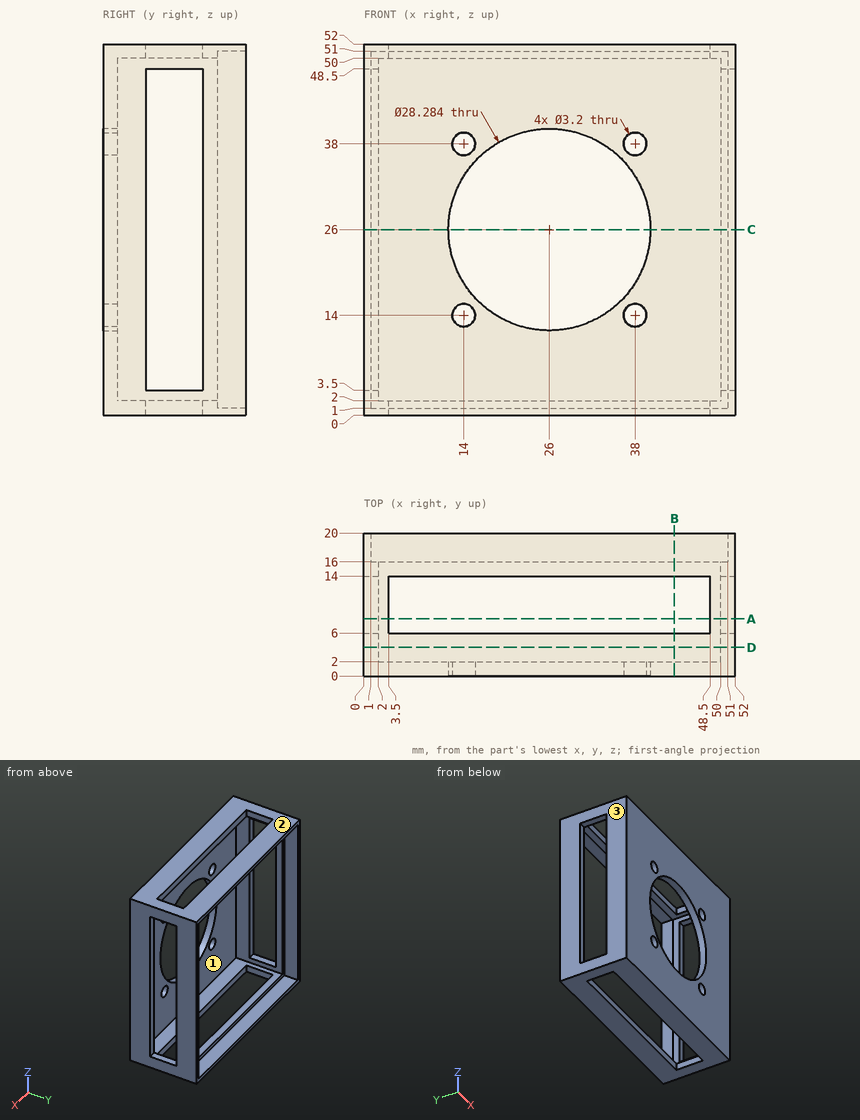
Here's the drawing with two shaded views (mm, measured from the low corner). I have some questions. Give positions to 0.01 mm unless a question says otherwise; leave off trailing zeros. Write each loop counter-clockwise with the first axis right and the second up, starting at its lowest first coordinate (ties: lowest second). Pieces come first, ordered by that corner, then holes. Notation, with made-up numbers: (46, 19.5) -> (95, 19.5) arc R23 cw to (95, 44.5) -> close; hole circle Ø7 at (3.5, -15.75). An arc over 180 degrees is marked (long way). One line per item, written item: value.
Q1. For P1, Ø15, axis at x = 14, z = 14.5, coming from the +Y side; P2, Ø1.9, axis at x = 14, z = 14, coming from the -Y side, each with a flat end and sliding along its axis, tell me the tip position at first contact or that it passes through.
Results found:
P1: stops at y = 2
P2: passes through
Q2. Imagine slicing it at B-B on x = 43.5. Please give me the cut outline in (y, z), and give its area (3 significant figures).
Results found:
outline: (0, 0) -> (6, 0) -> (6, 2) -> (2, 2) -> (2, 50) -> (6, 50) -> (6, 52) -> (0, 52) -> close; (14, 0) -> (20, 0) -> (20, 1) -> (16, 1) -> (16, 2) -> (14, 2) -> close; (14, 50) -> (16, 50) -> (16, 51) -> (20, 51) -> (20, 52) -> (14, 52) -> close
area: 136 mm^2
Q3. Imagine slicing it at D-D on y = 4. Please give me the cut outline in (x, z), and give its area (3 significant figures).
Results found:
outline: (0, 0) -> (52, 0) -> (52, 52) -> (0, 52) -> close; hole (2, 2) -> (50, 2) -> (50, 50) -> (2, 50) -> close
area: 400 mm^2
Q4. Imagine slicing it at C-C on z = 26. Please give me the cut outline in (x, y).
Results found:
outline: (0, 0) -> (11.86, 0) -> (11.86, 2) -> (2, 2) -> (2, 6) -> (0, 6) -> close; (0, 14) -> (2, 14) -> (2, 16) -> (1, 16) -> (1, 20) -> (0, 20) -> close; (40.14, 0) -> (52, 0) -> (52, 6) -> (50, 6) -> (50, 2) -> (40.14, 2) -> close; (50, 14) -> (52, 14) -> (52, 20) -> (51, 20) -> (51, 16) -> (50, 16) -> close
Q5. Imagine slicing it at A-A on y = 8. Please give me the cut outline in (x, z), and give its area (3 significant figures).
Results found:
outline: (0, 0) -> (3.5, 0) -> (3.5, 2) -> (2, 2) -> (2, 3.5) -> (0, 3.5) -> close; (0, 48.5) -> (2, 48.5) -> (2, 50) -> (3.5, 50) -> (3.5, 52) -> (0, 52) -> close; (48.5, 0) -> (52, 0) -> (52, 3.5) -> (50, 3.5) -> (50, 2) -> (48.5, 2) -> close; (48.5, 50) -> (50, 50) -> (50, 48.5) -> (52, 48.5) -> (52, 52) -> (48.5, 52) -> close
area: 40.0 mm^2
Q6. We'd pull the mould along Z, two halves only. Please class the marked faces 1, 2 and 3: +Z half, -Z half, draft (parallel to the pull), parting line (faces both ways), or undercut.
Results found:
face 1: undercut
face 2: +Z half
face 3: draft
Q7. Please list where these lines run through material, in increasing order: line 1 (X direction, y = 1.2, z = 26); line 2 (X direction, y = 1.2, z = 38) (1 decimal); line 3 (X direction, y = 4.5, z = 49). Write a range as [from, to].
Results found:
line 1: x = [0, 11.86], [40.14, 52]
line 2: x = [0, 12.4], [15.6, 18.5], [33.5, 36.4], [39.6, 52]
line 3: x = [0, 2], [50, 52]
